Model file for the job. Use its own axes, mm. A direction names the side the tool comes from. Round coordinates to 2 decimals unless told otherwise and drop trailing zeros. Write each loop counter-clockwise with the first axis right and the second up, starting at its lowest first coordinate (ties: lowest second). Pieces come first, ordered by that corner, then holes. Notation, with made-up numbers: (10, -35) - (45, -35) arc R14 cw to (45, -20) - close; hole circle Ø3 at (52.5, 3.25). An arc over 180 degrees is marked (long way). One line per item, written item: value.
from build123d import *

# Parameters (mm, degrees)
BOSS_EXTRUDE1_DEPTH = 18.5
SKETCH2_W           = 15
SKETCH2_H           = 48
CUT_EXTRUDE1_DEPTH  = 15
SKETCH3_R           = 1.75
CUT_EXTRUDE2_DEPTH  = 3.5
SKETCH4_R           = 1.75
CUT_EXTRUDE3_DEPTH  = 4
SKETCH5_R           = 1.75
CUT_EXTRUDE4_DEPTH  = 4
CUT_EXTRUDE5_DEPTH  = 19
FILLET1_R           = 2
FILLET2_R           = 5
FILLET3_R           = 1


with BuildPart() as part:
    # Sketch1 → Boss-Extrude1 (new body)
    with BuildSketch(Plane.XY):
        Polygon((20.545588903, 15.488794989), (48.258401824, -32.511205011), (7.85498998, -32.511205011), (-14.14501002, -32.511205011), (-14.14501002, 15.488794989), align=None)
    extrude(amount=BOSS_EXTRUDE1_DEPTH)

    # Sketch2 → Cut-Extrude1 (cut)
    with BuildSketch(Plane.XY):
        with Locations((-3.14501002, -8.511205011)):
            Rectangle(SKETCH2_W, SKETCH2_H)
        Polygon((44.21694994, -32.511205011), (19.886822921, 9.62981114), (6.896441864, 2.12981114), (26.896441864, -32.511205011), align=None)
    extrude(amount=CUT_EXTRUDE1_DEPTH, mode=Mode.SUBTRACT)

    # Sketch3 → Cut-Extrude2 (cut)
    with BuildSketch(Plane(origin=(22.116036645, 12.76869971, 0), x_dir=(0, 0, -1), z_dir=(0.8660254037844378, 0.5000000000000016, 0))):
        with Locations(Location((-7.5, -37.764004417, 0), (0, 0, 90))):
            Circle(SKETCH3_R)
        with Locations(Location((-7.5, -14.103750379, 0), (0, 0, 90))):
            Circle(SKETCH3_R)
    extrude(amount=-CUT_EXTRUDE2_DEPTH, mode=Mode.SUBTRACT)

    # Sketch4 → Cut-Extrude3 (cut)
    with BuildSketch(Plane(origin=(0, 0, 18.5), x_dir=(-1, 0, 0), z_dir=(0, 0, -1))):
        with Locations(Location((-29.306695902, -21.685887464, 0), (0, 0, 180))):
            Circle(SKETCH4_R)
        with Locations(Location((-19.641632393, -4.945506407, 0), (0, 0, 180))):
            Circle(SKETCH4_R)
        with Locations(Location((3.14501002, 2.988794989, 0), (0, 0, 180))):
            Circle(SKETCH4_R)
        with Locations(Location((3.14501002, -20.011205011, 0), (0, 0, 180))):
            Circle(SKETCH4_R)
    extrude(amount=CUT_EXTRUDE3_DEPTH, mode=Mode.SUBTRACT)

    # Sketch5 → Cut-Extrude4 (cut)
    with BuildSketch(Plane.ZY.offset(14.14501002)):
        with Locations(Location((7.5, -20.011205011, 0), (0, 0, 270))):
            Circle(SKETCH5_R)
        with Locations(Location((7.5, 2.988794989, 0), (0, 0, 270))):
            Circle(SKETCH5_R)
    extrude(amount=-CUT_EXTRUDE4_DEPTH, mode=Mode.SUBTRACT)

    # Sketch6 → Cut-Extrude5 (cut)
    with BuildSketch(Plane.XY.offset(18.5)):
        Polygon((44.21694994, -32.511205011), (47.248038853, -30.761205011), (48.258401824, -32.511205011), align=None)
    extrude(amount=-CUT_EXTRUDE5_DEPTH, mode=Mode.SUBTRACT)

    # Fillet1
    fillet1_edges = [part.edges().sort_by_distance(p)[0] for p in [
        (47.248038853, -30.761205011, 9.25),
    ]]
    fillet(fillet1_edges, radius=FILLET1_R)

    # Fillet2
    fillet2_edges = [part.edges().sort_by_distance(p)[0] for p in [
        (20.545588903, 15.488794989, 9.25),
    ]]
    fillet(fillet2_edges, radius=FILLET2_R)

    # Fillet3
    fillet3_edges = [part.edges().sort_by_distance(p)[0] for p in [
        (44.866468993, -32.136205011, 0),
        (46.447839698, -30.546792294, 0),
        (11.006913769, 15.488794989, 0),
        (20.158837557, 14.818922008, 0),
        (44.866468993, -32.136205011, 18.5),
        (46.447839698, -30.546792294, 18.5),
        (1.756913769, 15.488794989, 18.5),
        (20.158837557, 14.818922008, 18.5),
        (-14.14501002, 15.488794989, 9.25),
        (-14.14501002, -32.511205011, 9.25),
        (-14.14501002, -8.511205011, 0),
        (15.625715922, -32.511205011, 0),
        (4.35498998, -8.511205011, 0),
        (34.118501715, -8.020179607, 0),
        (-14.14501002, -8.511205011, 18.5),
        (15.03596996, -32.511205011, 18.5),
        (34.118501715, -8.020179607, 18.5),
    ]]
    fillet(fillet3_edges, radius=FILLET3_R)


solid = part.part
1. Drop flat-ended pins along their axis: pin 1 (4.5 mm diameter, centred on x = -2.5, y = -4.5, fed in from -Z); pin 2 (5.5 mm diameter, centred on y = -20.01, z = 7.5, fed in from +X); pin 3 (8 mm diameter, centred on x = 36, z = 2.5, fed in from -Y). Give the stop position or say it passes through.
Report:
pin 1: z = 15
pin 2: x = 42.63
pin 3: y = -25.21
2. Mould opens along Y. For faces 4 (the face through (-10.645, -9, 7)), 5 (the face through (44.7, -31.9, 18.2)), 6 (the face through (25, -11, 15)), 7 (the face through (33.95, -7.73, 9.13)) say: released by +Y, released by -Y, zero draft, split by the parting line, or undercut.
Report:
face 4: zero draft
face 5: released by -Y
face 6: undercut
face 7: released by +Y
3. Band-saw the part on B-B on x = -7. Write the cut outline in (y, z).
Report:
outline: (-32.51, 15) - (15.49, 15) - (15.49, 17.5) arc R1 ccw to (14.49, 18.5) - (-31.51, 18.5) arc R1 ccw to (-32.51, 17.5) - close
4. Band-saw the part on C-C on z = 7.5. State how many separate pieces and enclosed holes the cut face has, plus the area to 3 significant figures.
Report:
separate pieces: 6
enclosed holes: 0
area: 890 mm²
5. Band-saw the part on A-A on z = 11.25. Write the cut outline in (x, y).
Report:
outline: (-14.15, -31.51) arc R1 ccw to (-13.15, -32.51) - (-10.65, -32.51) - (-10.65, 15.49) - (-13.15, 15.49) arc R1 ccw to (-14.15, 14.49) - close; (4.35, -32.51) - (26.9, -32.51) - (6.9, 2.13) - (19.89, 9.63) - (44.22, -32.51) - (45.52, -31.76) arc R2 ccw to (46.25, -29.03) - (21.99, 12.99) arc R5 ccw to (17.66, 15.49) - (4.35, 15.49) - close
6. Tool access for faces 1 (the face through (-12.42, -21.63, 6.83)), 2 (the face through (4.355, -9, 8)), 3 (the face through (32.2, -11.7, 7.4)): list every direction of +Z, -Z, +X, -X, +Y, -Y with a clear straight run to the whole face (end or side of a thin tool).
Report:
face 1: -X
face 2: -Z, +Y, -Y
face 3: -Z
7. Wall check: probe 1 along X at (y, z) = (9, 5.5); probe 2 along X at (y, z) = (-14.5, 6); probe 3 along Z at (x, y) = (16.5, -8.5). Give the ranges that are in metal, low to high. Write a range as [from, to].
Report:
probe 1: [-14.15, -10.65], [4.35, 18.8], [20.25, 24.29]
probe 2: [-14.15, -10.65], [4.35, 16.5], [33.82, 37.86]
probe 3: [15, 18.5]
